Geometry check sheet. Reference: the model listing, model coordinates, mm. A direction names the side the tool comes from. Coordinates: 2 decimals unless noted, no trailing zeros. Loops run counter-clockwise (first coordinate to the right, second up) from the corner with the lowest first, then second, coordinate; pieces in that order, holes last. Notation, with made-up numbers: (75, 3) -> (124, 3) arc R29 ccw to (124, 41) -> close; hole circle Ø4 at (43.5, 40.25). An arc over 180 degrees is marked (long way). Answer as a JSON object with one key per item and string values.
from build123d import *

# Parameters (mm, degrees)
SKETCH1_R           = 6.35
BOSS_EXTRUDE1_DEPTH = 81
CUT_EXTRUDE1_START  = -75.2
SKETCH2_R           = 12.7
SKETCH2_R_2         = 5.715
CUT_EXTRUDE1_DEPTH  = 1.016
BOSS_EXTRUDE2_START = -67
SKETCH3_R           = 8.89
BOSS_EXTRUDE2_DEPTH = 3
SKETCH4_R           = 7.62
SKETCH4_R_2         = 5.08
CUT_EXTRUDE2_DEPTH  = 6.35
CUT_EXTRUDE4_START  = -17.5
SKETCH5_R           = 12.7
SKETCH5_R_2         = 5.715
CUT_EXTRUDE4_DEPTH  = 1
CUT_EXTRUDE5_START  = -45
SKETCH6_R           = 12.7
SKETCH6_R_2         = 5.715
CUT_EXTRUDE5_DEPTH  = 1


with BuildPart() as part:
    # Sketch1 → Boss-Extrude1 (new body)
    with BuildSketch(Plane.XY):
        Circle(SKETCH1_R)
    extrude(amount=-BOSS_EXTRUDE1_DEPTH)

    # Sketch2 → Cut-Extrude1 (cut)
    with BuildSketch(Plane.XY.offset(CUT_EXTRUDE1_START)):
        with Locations((0.049037486, 0)):
            Circle(SKETCH2_R)
        Circle(SKETCH2_R_2, mode=Mode.SUBTRACT)
    extrude(amount=-CUT_EXTRUDE1_DEPTH, mode=Mode.SUBTRACT)

    # Sketch3 → Boss-Extrude2 (add)
    with BuildSketch(Plane.XY.offset(BOSS_EXTRUDE2_START)):
        Circle(SKETCH3_R)
    extrude(amount=BOSS_EXTRUDE2_DEPTH)

    # Sketch4 → Cut-Extrude2 (cut)
    with BuildSketch(Plane.XY):
        Circle(SKETCH4_R)
        Circle(SKETCH4_R_2, mode=Mode.SUBTRACT)
    extrude(amount=-CUT_EXTRUDE2_DEPTH, mode=Mode.SUBTRACT)

    # Sketch5 → Cut-Extrude4 (cut)
    with BuildSketch(Plane.XY.offset(CUT_EXTRUDE4_START)):
        Circle(SKETCH5_R)
        Circle(SKETCH5_R_2, mode=Mode.SUBTRACT)
    extrude(amount=-CUT_EXTRUDE4_DEPTH, mode=Mode.SUBTRACT)

    # Sketch6 → Cut-Extrude5 (cut)
    with BuildSketch(Plane.XY.offset(CUT_EXTRUDE5_START)):
        Circle(SKETCH6_R)
        Circle(SKETCH6_R_2, mode=Mode.SUBTRACT)
    extrude(amount=-CUT_EXTRUDE5_DEPTH, mode=Mode.SUBTRACT)


solid = part.part
1. Thickness scan on probe 1 along Z at (x, y) = (-5.75, 0.25); probe 2 along Z at (x, y) = (-7, -5); probe 3 along X at (y, z) = (2.75, -27). Record the ranges inside material, lowest first. Write a range as from..to.
Evaluation:
{"probe 1": "z = -81..-76.22, -75.2..-46, -45..-18.5, -17.5..-6.35", "probe 2": "z = -67..-64", "probe 3": "x = -5.72..5.72"}
2. Section check A-A, the plane z = -8. Record the boundary of the cut face in (x, y).
Evaluation:
{"outline": "circle Ø12.7 at (0, 0)"}
3. Tool access check on faces 1 (the face through (-1.38, -6.2, -31.56)), 2 (the face through (-1.38, -6.2, -78.57)), 3 (the face through (-6, 1, -46)). Record the directions out of +Z, -Z, +X, -X, +Y, -Y that give a thin tool (end or side, any length) a straight path to the whole face; none if there is none.
Evaluation:
{"face 1": "+Z", "face 2": "-Z", "face 3": "none"}
4. Depth check by flat-ended pin: P1, Ø1.5, axis at y = -2, z = -54, coming from the -X side; P2, Ø4, axis at y = -2, z = -55, coming from the +X side; P3, Ø6, axis at x = 5.5, z = -30, coming from the +Y side. Enter the tip coordinate at first touch or a pass-through.
Evaluation:
{"P1": "stops at x = -6.23", "P2": "stops at x = 6.35", "P3": "stops at y = 5.84"}
5. Section check B-B, the plane z = -66. Record the boundary of the cut face in (x, y), then the cut area to 3 significant figures.
Evaluation:
{"outline": "circle Ø17.78 at (0, 0)", "area": "248 mm^2"}
6. Mould release check, pull along Z, two halves, no side actions. Record for faces 4 (the face through (2, 5, -6.35)), 5 (the face through (-6, 1, -76.216)), 6 (the face through (-1.38, -6.2, -54.87)): released by +Z, released by -Z, zero draft, split by the parting line, or undercut.
Evaluation:
{"face 4": "released by +Z", "face 5": "undercut", "face 6": "zero draft"}
